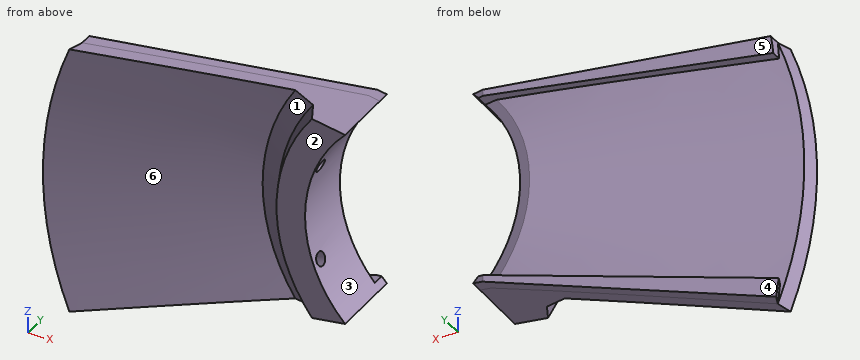
from build123d import *

# Parameters (mm, degrees)
RIVOLUZIONE1_ANGLE                 = 44
RIVOLUZIONE1_OTHER_WAY_ANGLE       = 44
TAGLIO_ESTRUSIONE1_DEPTH           = 59
FORO_PER_VITE_M4_1_D               = 5.6
FORO_PER_VITE_M4_1_DEPTH           = 8.1
FORO_PER_VITE_M4_1_TIP             = 1.682409733
FORO_PER_VITE_M4_1_ON_FACE_2_D     = 5.6
FORO_PER_VITE_M4_1_ON_FACE_2_DEPTH = 8.1
FORO_PER_VITE_M4_1_ON_FACE_2_TIP   = 1.682409733
RIVOLUZIONE2_ANGLE                 = 3
RIVOLUZIONE3_ANGLE                 = 3
TAGLIO_ESTRUSIONE2_START           = -59
SCHIZZO7_R                         = 60
TAGLIO_ESTRUSIONE2_DEPTH           = 59


with BuildPart() as part:
    # Schizzo1 → Rivoluzione1 (revolve)
    with BuildSketch(Plane(origin=(0, 0, 0), x_dir=(-1, 0, 0), z_dir=(0, 0, -1))):
        Polygon((83.801322108, 10.249602265), (156.30594507, -23.559858674), (154.630778704, -17.261826174), (64, 25), (60, 25), (60, 0), (72, 0), (75.34408852, 7.171420975), align=None)
    revolve(axis=Axis((0, 0, 0), (0, 1, 0)), revolution_arc=RIVOLUZIONE1_ANGLE)

    # Schizzo1 → Rivoluzione1 other way (revolve)
    with BuildSketch(Plane(origin=(0, 0, 0), x_dir=(-1, 0, 0), z_dir=(0, 0, -1))):
        Polygon((83.801322108, 10.249602265), (156.30594507, -23.559858674), (154.630778704, -17.261826174), (64, 25), (60, 25), (60, 0), (72, 0), (75.34408852, 7.171420975), align=None)
    revolve(axis=Axis((0, 0, 0), (0, -1, 0)), revolution_arc=RIVOLUZIONE1_OTHER_WAY_ANGLE)

    # Schizzo6 → Taglio-Estrusione1 (cut)
    with BuildSketch(Plane(origin=(0, 25, 0), x_dir=(1, 0, 0), z_dir=(0, 1, 0))):
        with BuildLine():
            Line((-43.16038802, 41.679502228), (-145.209485409, 57.842491403))
            ThreePointArc((-145.209485409, 57.842491403), (-131.297347075, 84.808932993), (-112.437087319, 108.579233096))
            Line((-112.437087319, 108.579233096), (-43.16038802, 41.679502228))
        make_face()
        with BuildLine():
            Line((-43.16038802, -41.679502228), (-145.209485409, -57.842491403))
            ThreePointArc((-145.209485409, -57.842491403), (-131.297347075, -84.808932993), (-112.437087319, -108.579233096))
            Line((-112.437087319, -108.579233096), (-43.16038802, -41.679502228))
        make_face()
    extrude(amount=-TAGLIO_ESTRUSIONE1_DEPTH, mode=Mode.SUBTRACT)

    # Foro per Vite M4-1
    with Locations(Plane(origin=(-56.381557247, 5, 20.5212086), x_dir=(0.342020143326, 0, 0.939692620786), z_dir=(0.939692620786, 0, -0.342020143326))):
        with Locations((0, 0)):
            Hole(FORO_PER_VITE_M4_1_D / 2, depth=FORO_PER_VITE_M4_1_DEPTH)
            with Locations((0, 0, -(FORO_PER_VITE_M4_1_DEPTH + FORO_PER_VITE_M4_1_TIP / 2))):  # 118° drill point
                Cone(0, FORO_PER_VITE_M4_1_D / 2, FORO_PER_VITE_M4_1_TIP, mode=Mode.SUBTRACT)

    # Foro per Vite M4-1 on face 2
    with Locations(Plane(origin=(-56.381557247, 5.000002473, -20.5212086), x_dir=(-0.342019894889, 0, 0.939692711209), z_dir=(0.939692711209, 0, 0.342019894889))):
        with Locations((0, 0)):
            Hole(FORO_PER_VITE_M4_1_ON_FACE_2_D / 2, depth=FORO_PER_VITE_M4_1_ON_FACE_2_DEPTH)
            with Locations((0, 0, -(FORO_PER_VITE_M4_1_ON_FACE_2_DEPTH + FORO_PER_VITE_M4_1_ON_FACE_2_TIP / 2))):  # 118° drill point
                Cone(0, FORO_PER_VITE_M4_1_ON_FACE_2_D / 2, FORO_PER_VITE_M4_1_ON_FACE_2_TIP, mode=Mode.SUBTRACT)

    # Schizzo2 → Rivoluzione2 (revolve)
    with BuildSketch(Plane(origin=(7.537525881, 0, -33.649741509), x_dir=(-0.9876883405951378, 0, -0.15643446504023117), z_dir=(0.15643446504023117, 0, -0.9876883405951378))):
        Polygon((51.329869775, 25), (51.329869775, 30), (55.329869775, 30), (154.933952788, -12.679561819), (152.933239569, -17.261826174), (56.140326971, 25), align=None)
    revolve(axis=Axis((5.383627379, 0, -33.990885517), (0, 1, 0)), revolution_arc=RIVOLUZIONE2_ANGLE)

    # Schizzo3 → Rivoluzione3 (revolve)
    with BuildSketch(Plane(origin=(7.537525881, 0, 33.649741509), x_dir=(0.9876883405951378, 0, -0.15643446504023112), z_dir=(0.15643446504023112, 0, 0.9876883405951378))):
        Polygon((-51.329869775, 25), (-56.140326971, 25), (-152.933239569, -17.261826174), (-152.933239569, -12.261826174), (-55.329869775, 30), (-51.329869775, 30), align=None)
    revolve(axis=Axis((5.383627379, 0, 33.990885517), (0, -1, 0)), revolution_arc=RIVOLUZIONE3_ANGLE)

    # Schizzo7 → Taglio-Estrusione2 (cut)
    with BuildSketch(Plane(origin=(0, 30, 0), x_dir=(1, 0, 0), z_dir=(0, 1, 0)).offset(TAGLIO_ESTRUSIONE2_START)):
        Circle(SCHIZZO7_R)
    extrude(amount=TAGLIO_ESTRUSIONE2_DEPTH, mode=Mode.SUBTRACT)


solid = part.part
For this review, take the finished solid that the model builds, in its own axes (mm). Face numbers are marked on the shaded views. A direction names the side the tool comes from. Coordinates: 2 decimals unless noted, no trailing zeros. Loops run counter-clockwise (first coordinate to the right, second up) from the corner with the lowest first, then second, coordinate; pieces in that order, holes last. Notation, with made-up numbers: (-20.5, 7.25) -> (13.5, 7.25) arc R20 cw to (13.5, 13.25) -> close; hole circle Ø3 at (28.5, -6.5). An arc over 180 degrees is marked (long way). Write each question's results on one line, items separated by ' | '.
Q1. To check wall thickness, follow line 1 along X through (y, z) = (7, -31.5); line 2 along X through (y, z) = (-7.5, 26.5); line 3 along X through (y, z) = (23, -3.5). State the ranges of each line that lie inside material, in increasing order. Write a range as [from, to].
Taken from the geometry:
line 1: [-97.65, -85.13], [-68.36, -51.07] | line 2: [-131.04, -118.95] | line 3: [-68.2, -59.9]
Q2. Add section D-D, the plane y = -1.5. State the section outline as (x, z) points.
Taken from the geometry:
outline: (-120.59, -47.23) arc R126.66 ccw to (-119.72, -53.81) -> (-96.77, -50.17) arc R109 cw to (-96.77, 50.17) -> (-118.96, 53.69) arc R125.9 ccw to (-119.82, 47.15) -> (-111.61, 46.29) arc R120.83 ccw to (-111.61, -46.29) -> close
Q3. Add section A-A, the plane y = 27.5. State the section outline as (x, z) points.
Taken from the geometry:
outline: (-53.28, -40.16) arc R58.98 ccw to (-52.87, -43.22) -> (-43.16, -41.68) arc R60 cw to (-45.32, -39.32) -> close; (-53.22, 40.15) -> (-45.32, 39.32) arc R60 cw to (-43.16, 41.68) -> (-52.81, 43.21) arc R58.92 ccw to start
Q4. Machinability: for the marked faces 5 and 6, which of the approach directions +Z, -Z, +X, -X, +Y, -Y give a long, thin tool a straight path to every point of the face, cutting with its end or side? Answer none if there is none.
Taken from the geometry:
face 5: +Z, -X, +Y | face 6: -Y
Q5. Mouldability with a two-part tool opening along X and no side actions: class the marked faces 1, 2, 3 and 4 as +X half, -X half, draft (parallel to the pull), parting line (faces both ways), or undercut.
Taken from the geometry:
face 1: undercut | face 2: draft | face 3: +X half | face 4: -X half
Q6. Add section C-C, the plane y = -9. State the section outline as (x, z) points.
Taken from the geometry:
outline: (-137.99, -49.06) arc R144.17 ccw to (-137.01, -56.54) -> (-113.39, -52.8) arc R125.08 cw to (-113.39, 52.8) -> (-136.07, 56.4) arc R143.22 ccw to (-137.05, 48.96) -> (-128.21, 48.03) arc R136.91 ccw to (-128.21, -48.03) -> close
Q7. Add section B-B, the plane z = 0. State the section outline as (x, y) points.
Taken from the geometry:
outline: (-156.31, -23.56) -> (-83.8, 10.25) -> (-75.34, 7.17) -> (-72, 0) -> (-60, 0) -> (-60, 25) -> (-64, 25) -> (-154.63, -17.26) -> close
Q8. For pin 1 Ø1.5 at (x, y) = (-138, -12.5) entering from +Z; pin 2 Ø1.5 at (y, z) = (7, -43) entering from -X; pin 3 Ø3 at (x, z) = (-136, 34) entering from +Y, all flat-tipped, find the tip position at first contact; note any pin that passes through.
Taken from the geometry:
pin 1: z = 56.82 | pin 2: x = -94.96 | pin 3: y = -9.83
